Check sheet for the modelled part. Datum: model origin and axes. Units: mm. A direction names the side the tool comes from. Coordinates: 2 decimals unless noted, no trailing zeros. Order: outer loops, then holes, each group sorted by start corner. A loop starts at its lowest first (then second) coordinate and runs counter-clockwise, first axis right, second up.
1. Set-up check for faces 1 (the flat face through (1, -3.175, 38)), 2 (the flat face through (14.288, 9, 55)), 3 (the flat face through (38.1, -1, 27)), 4 (the flat face through (-1, 35, 19.05)), 5 (the flat face through (-1, -47.625, 9)): record each of +Z, -Z, +X, -X, +Y, -Y from which the full face is reachable in a straight line by a thin tool's end or side.
2. Draft check along X on faces 6 (the flat face through (0, 9, 41.275)), 7 (the flat face through (-14.288, 9, 55)), 8 (the flat face through (-38.1, -1, 27)), 9 (the flat face through (26, 9, 69.85)). Enter one of: released by +X, released by -X, zero draft, split by the parting line, or undercut.
3. Thickness scan on line 1 (X direction, y = 15.5, z = 42); line 2 (Y direction, x = -9, z = 27) (3 decimals); line 3 (Z direction, x = -12.5, y = -38.5). Record the ranges inside material, lowest first.
4. Gauge pin test, flat ends, axial feed: pin 1 Ø13.5 at (x, y) = (0.5, -18.5) entering from +Z; pin 2 Ø6 at (x, z) = (5.5, 40) entering from -Y (3 decimals); pin 3 Ø7.5 at (x, y) = (2, 15) entering from +Z (3 decimals). Record the tip position at first contact, or that the pin passes through.
5. Cross-section at A-A (z = 48.5). Enter the section's corners in (x, y) (1 decimal).
6. Cross-section at C-C (x = 9.5). Enter the section's corners in (y, z) (3 decimals), then the cut area to 3 significant figures.
7. Cross-section at D-D (z = 25). Enter the section's corners in (x, y) (3 decimals).
```python
from build123d import *

# Parameters (mm, degrees)
F0_W     = 76.2
F0_H     = 95.25
F1_DEPTH = 19.05
F2_W     = 25.4
F2_H     = 50.8
F3_DEPTH = 76.2
F6_W     = 28.575
F6_H     = 28.575
F7_DEPTH = 127


with BuildPart() as f1:
    # F0 (on Top) → F1 (new body)
    with BuildSketch(Plane.XY):
        Rectangle(F0_W, F0_H)
    extrude(amount=F1_DEPTH)

    # F2 (on face) → F3 (join, through all)
    with BuildSketch(Plane.YZ.offset(38.1)):
        with Locations((9.525, 44.45)):
            Rectangle(F2_W, F2_H)
    extrude(amount=-F3_DEPTH)

    # F6 (on face) → F7 (cut)
    with BuildSketch(Plane.XZ.offset(3.175)):
        with Locations((0, 55.5625)):
            Rectangle(F6_W, F6_H)
    extrude(amount=-F7_DEPTH, mode=Mode.SUBTRACT)


solid = f1.part
```
Data:
1. face 1: +Z, +X, -X, -Y
1. face 2: +Z, +Y, -Y
1. face 3: +Z, -Z, +X, +Y, -Y
1. face 4: +Z, +X, -X, +Y
1. face 5: +Z, -Z, +X, -X, -Y
2. face 6: undercut
2. face 7: undercut
2. face 8: released by -X
2. face 9: zero draft
3. line 1: x = -38.1 to -14.29, 14.29 to 38.1
3. line 2: y = -3.175 to 22.225
3. line 3: z = 0 to 19.05
4. pin 1: stops at z = 19.05
4. pin 2: stops at y = -3.175
4. pin 3: stops at z = 41.275
5. outline: (-38.1, -3.2) - (-14.3, -3.2) - (-14.3, 22.2) - (-38.1, 22.2) - close; (14.3, -3.2) - (38.1, -3.2) - (38.1, 22.2) - (14.3, 22.2) - close
6. outline: (-47.625, 0) - (47.625, 0) - (47.625, 19.05) - (22.225, 19.05) - (22.225, 41.275) - (-3.175, 41.275) - (-3.175, 19.05) - (-47.625, 19.05) - close
6. area: 2,380 mm2
7. outline: (-38.1, -3.175) - (38.1, -3.175) - (38.1, 22.225) - (-38.1, 22.225) - close
